from build123d import *

# Parameters (mm, degrees)
SKETCH1_R           = 40
SKETCH1_R_2         = 12.5
BOSS_EXTRUDE1_DEPTH = 3
BOSS_EXTRUDE5_DEPTH = 10
SKETCH20_R          = 1.5
CUT_EXTRUDE3_DEPTH  = 5
SKETCH22_R          = 1.5
CUT_EXTRUDE4_DEPTH  = 10
CIRPATTERN1_COUNT   = 3
SKETCH24_R          = 1.5
CUT_EXTRUDE5_DEPTH  = 10
CIRPATTERN2_COUNT   = 3


with BuildPart() as part:
    # Sketch1 → Boss-Extrude1 (new body)
    with BuildSketch(Plane(origin=(0, 0, 0), x_dir=(1, 0, 0), z_dir=(0, 1, 0))):
        with Locations(Location((0, 0, 0), (0, 0, 270))):
            Circle(SKETCH1_R)
        with Locations(Location((0, 0, 0), (0, 0, 270))):
            Circle(SKETCH1_R_2, mode=Mode.SUBTRACT)
    extrude(amount=BOSS_EXTRUDE1_DEPTH)

    # Sketch8 → Boss-Extrude5 (add)
    with BuildSketch(Plane(origin=(0, 3, 0), x_dir=(1, 0, 0), z_dir=(0, 1, 0))):
        with BuildLine():
            Line((-4, -39.799497484), (-4, -28.466262232))
            Line((-4, -28.466262232), (-9, -28.466262232))
            Line((-9, -28.466262232), (-9, -38.97435054))
            ThreePointArc((-9, -38.97435054), (-6.513080444, -39.466185313), (-4, -39.799497484))
        make_face()
        with BuildLine():
            Line((4, -28.466262232), (4, -39.799497484))
            ThreePointArc((4, -39.799497484), (6.513080444, -39.466185313), (9, -38.97435054))
            Line((9, -38.97435054), (9, -28.466262232))
            Line((9, -28.466262232), (4, -28.466262232))
        make_face()
    boss_extrude5 = extrude(amount=BOSS_EXTRUDE5_DEPTH)

    # Sketch9 for Loft4 → Loft4 section 0
    with BuildSketch(Plane(origin=(9, 0, 0), x_dir=(0, 0, -1), z_dir=(1, 0, 0))):
        with BuildLine():
            Line((-28.466262232, 13), (-38.97435054, 13))
            # circular arc as an exact rational Bezier (weights 1, cos(half-angle), 1)
            Bezier((-38.97435054, 13), (-33.720306386, 30.574863042), (-28.466262232, 13), weights=[1, 0.286426753, 1])
        make_face()
    # Sketch10 for Loft4 → Loft4 section 1
    with BuildSketch(Plane.ZY.offset(-4)):
        with BuildLine():
            Line((28.466262232, 13), (39.799497484, 13))
            Bezier((39.799497484, 13), (34.132879858, 28.686313092), (28.466262232, 13), weights=[1, 0.339756679, 1])
        make_face()
    loft4 = loft()

    # Loft7: read off the stored shape, not the designer's step
    # Loft7: loft between two sections, ruled curve by curve
    loft7_from = [
        Edge.make_bspline([(-4, 13, 39.799497484), (-4, 13.445887075, 39.644015382), (-4, 13.912406496, 39.42235746), (-4, 14.83103025, 38.804929607), (-4, 15.282819738, 38.407898984), (-4, 16.078747391, 37.428773866), (-4, 16.421172618, 36.845868146), (-4, 16.895486355, 35.552548175), (-4, 17.025283738, 34.843378132), (-4, 17.025283738, 33.422381584), (-4, 16.895486355, 32.713211541), (-4, 16.421172618, 31.419891571), (-4, 16.078747391, 30.83698585), (-4, 15.282819738, 29.857860733), (-4, 14.83103025, 29.460830109), (-4, 13.912406496, 28.843402256), (-4, 13.445887075, 28.621744334), (-4, 13, 28.466262232)], [0, 0, 0, 0, 0.125, 0.125, 0.25, 0.25, 0.375, 0.375, 0.5, 0.5, 0.625, 0.625, 0.75, 0.75, 0.875, 0.875, 1, 1, 1, 1], 3),
        Edge.make_line((-4, 13, 28.466262232), (-4, 13, 39.799497484)),
    ]
    loft7_to = [
        Edge.make_bspline([(-9, 13, 38.97435054), (-9, 13.419469841, 38.848866269), (-9, 13.863009903, 38.66161005), (-9, 14.746425178, 38.117380283), (-9, 15.186117881, 37.75901052), (-9, 15.967952584, 36.854602056), (-9, 16.308267994, 36.307496065), (-9, 16.781693902, 35.08000068), (-9, 16.912355403, 34.400917098), (-9, 16.912355403, 33.039695674), (-9, 16.781693902, 32.360612092), (-9, 16.308267994, 31.133116706), (-9, 15.967952584, 30.586010716), (-9, 15.186117881, 29.681602252), (-9, 14.746425178, 29.323232488), (-9, 13.863009903, 28.779002722), (-9, 13.419469841, 28.591746503), (-9, 13, 28.466262232)], [0, 0, 0, 0, 0.125, 0.125, 0.25, 0.25, 0.375, 0.375, 0.5, 0.5, 0.625, 0.625, 0.75, 0.75, 0.875, 0.875, 1, 1, 1, 1], 3),
        Edge.make_line((-9, 13, 28.466262232), (-9, 13, 38.97435054)),
    ]
    loft7 = Solid(Shell([*[Face.make_surface_from_curves(loft7_from[k], loft7_to[k]) for k in range(2)], Face(Wire(loft7_from)), Face(Wire(loft7_to))]))
    add(loft7)

    # Sketch20 → Cut-Extrude3 (cut)
    with BuildSketch(Plane.ZY.offset(-4)):
        with Locations((34.132879858, 13)):
            Circle(SKETCH20_R)
    cut_extrude3 = extrude(amount=-CUT_EXTRUDE3_DEPTH, mode=Mode.SUBTRACT)

    # Sketch22 → Cut-Extrude4 (cut)
    with BuildSketch(Plane(origin=(-4, 0, 0), x_dir=(0, 0, -1), z_dir=(1, 0, 0))):
        with Locations((-34.090737301, 12.972785767)):
            Circle(SKETCH22_R)
    cut_extrude4 = extrude(amount=-CUT_EXTRUDE4_DEPTH, mode=Mode.SUBTRACT)

    # CirPattern1: Boss-Extrude5, Loft4, Loft7, Cut-Extrude3, Cut-Extrude4 ×3 about axis
    cirpattern1_axis = Axis((0, 0, 0), (0, 1, 0))
    add([boss_extrude5.rotate(cirpattern1_axis, i * 360 / CIRPATTERN1_COUNT) for i in range(1, CIRPATTERN1_COUNT)])
    add([loft4.rotate(cirpattern1_axis, i * 360 / CIRPATTERN1_COUNT) for i in range(1, CIRPATTERN1_COUNT)])
    add([loft7.rotate(cirpattern1_axis, i * 360 / CIRPATTERN1_COUNT) for i in range(1, CIRPATTERN1_COUNT)])
    add([cut_extrude3.rotate(cirpattern1_axis, i * 360 / CIRPATTERN1_COUNT) for i in range(1, CIRPATTERN1_COUNT)], mode=Mode.SUBTRACT)
    add([cut_extrude4.rotate(cirpattern1_axis, i * 360 / CIRPATTERN1_COUNT) for i in range(1, CIRPATTERN1_COUNT)], mode=Mode.SUBTRACT)

    # Sketch24 → Cut-Extrude5 (cut)
    with BuildSketch(Plane(origin=(0, 3, 0), x_dir=(1, 0, 0), z_dir=(0, 1, 0))):
        with Locations(Location((29.444863729, -17, 0), (0, 0, 270))):
            Circle(SKETCH24_R)
    cut_extrude5 = extrude(amount=-CUT_EXTRUDE5_DEPTH, mode=Mode.SUBTRACT)

    # CirPattern2: Cut-Extrude5 ×3 about axis
    cirpattern2_axis = Axis((0, 0, 0), (0, 1, 0))
    for i in range(1, CIRPATTERN2_COUNT):
        add(cut_extrude5.rotate(cirpattern2_axis, i * 360 / CIRPATTERN2_COUNT), mode=Mode.SUBTRACT)


solid = part.part
Verification items for the finished model (mm, model axes). A direction names the side the tool comes from. Round coordinates to 2 decimals unless told otherwise and drop trailing zeros. Loops run counter-clockwise (first coordinate to the right, second up) from the corner with the lowest first, then second, coordinate; pieces in that order, holes last. Notation, with made-up numbers: (-3, 52.25) - (56, 52.25) arc R26 ccw to (56, 77.25) - close; hole circle Ø1 at (35, 71.25). An arc over 180 degrees is marked (long way). Use a Markdown table: item, result. Add a question column.
1. Section check C-C, the plane z = 0. Record the boundary of the cut face in (x, y), plus the area to 3 significant figures.
2. Access from +Z, -Z, +X, -X, +Y, -Y to the whole of each face (thin tool, end or side, straight path). Record for faces 4 (the face through (-24.64, 9.86, -24.62)), 5 (the face through (4, 10, 34)), 6 (the face through (-6, 8, 28.466)).
3. Section check D-D, the plane y = 1.25. Record the boundary of the cut face in (x, z), plus the area to 3 significant figures.
4. Release check for a two-part mould opening along X. For faces 1 (the face through (7, 8, 28.466)), 2 (the face through (27.49, 10.31, -20.49)), 3 (the face through (-28.99, 1.52, 18.43)) record: released by +X, released by -X, zero draft, split by the parting line, or undercut.
5. Thickness scan on probe 1 along X at (y, z) = (0.65, 0); probe 2 along X at (y, z) = (2, 17); probe 3 along Y at (x, z) = (-25, 9). Record the ranges inside material, lowest first. Write a range as [from, to].
6. Section check B-B, the plane y = 7.25. Record the boundary of the cut face in (x, z).
7. Gauge pin test, flat ends, axial feed: pin 1 (6 mm diameter, centred on y = 14, z = -5, fed in from +X); pin 2 (0.9 mm diameter, centred on x = 7, z = 39.5, fed in from +Y); pin 3 (4 mm diameter, centred on y = 12.97, z = 34.09, fed in from +X); pin 4 (1.8 mm diameter, centred on x = 29.44, z = 17, fed in from -Y). Record the tip position at first contact, or that the pin passes through.
8. Section check A-A, the plane x = 0. Record the boundary of the cut face in (y, z), plus the area to 3 significant figures.
Checks:
| question | item | result |
|---|---|---|
| 1 | outline | (-40, 0) - (-12.5, 0) - (-12.5, 3) - (-40, 3) - close; (12.5, 0) - (40, 0) - (40, 3) - (12.5, 3) - close |
| 1 | area | 165 mm^2 |
| 2 | face 4 | -Z, +Y |
| 2 | face 5 | +Z, -Z, +Y |
| 2 | face 6 | -Z, +X, -X, +Y |
| 3 | outline | circle Ø80 at (0, 0); hole circle Ø3 at (-29.44, 17); hole circle Ø25 at (0, 0); hole circle Ø3 at (0, -34); hole circle Ø3 at (29.44, 17) |
| 3 | area | 4,510 mm^2 |
| 4 | face 1 | zero draft |
| 4 | face 2 | released by +X |
| 4 | face 3 | undercut |
| 5 | probe 1 | x = [-40, -12.5], [12.5, 40] |
| 5 | probe 2 | x = [-36.21, -30.94], [-27.94, 27.94], [30.94, 36.21] |
| 5 | probe 3 | y = [0, 3] |
| 6 | outline | (-38.25, -11.69) arc R40 ccw to (-36.47, -16.44) - (-26.65, -10.77) - (-29.15, -6.44) - close; (-32.47, -23.36) arc R40 ccw to (-29.25, -27.28) - (-20.15, -22.03) - (-22.65, -17.7) - close; (-9, 28.47) - (-4, 28.47) - (-4, 39.8) arc R40 ccw to (-9, 38.97) - close; (4, 28.47) - (9, 28.47) - (9, 38.97) arc R40 ccw to (4, 39.8) - close; (20.15, -22.03) - (29.25, -27.28) arc R40 ccw to (32.47, -23.36) - (22.65, -17.7) - close; (26.65, -10.77) - (36.47, -16.44) arc R40 ccw to (38.25, -11.69) - (29.15, -6.44) - close |
| 7 | pin 1 | stops at x = 31.86 |
| 7 | pin 2 | stops at y = 13.66 |
| 7 | pin 3 | stops at x = 9 |
| 7 | pin 4 | passes through |
| 8 | outline | (0, -40) - (3, -40) - (3, -35.5) - (0, -35.5) - close; (0, -32.5) - (3, -32.5) - (3, -12.5) - (0, -12.5) - close; (0, 12.5) - (3, 12.5) - (3, 40) - (0, 40) - close |
| 8 | area | 156 mm^2 |
